The listing builds one solid part. Answer for the finished solid, in the listing's coordinates (mm). Round coordinates to 2 decimals unless told otherwise and drop trailing zeros. Write each loop counter-clockwise with the first axis right and the second up, starting at its lowest first coordinate (ties: lowest second). Pieces come first, ordered by that corner, then holes.
(1) The mould has two halves that part along Y. Classify faces 1 (the face through (21.403, 9.898, 1.479)), 2 (the face through (1, 2, 2)), 3 (the face through (73, 29, 2)): +Y half, -Y half, draft (parallel to the pull), parting line (faces both ways), or undercut.
(2) Each of these flat-tipped pins is pushed along its axis until it touches: pin 1 Ø9.5 at (x, y) = (16.4, 8.32) entering from +Z; pin 2 Ø4 at (x, y) = (23.5, 15) entering from -Z. Where does it stop, or does it pass through?
(3) Find the intervals of material crossed by probe 1 along X at (y, z) = (4.5, 2); probe 2 along X at (y, z) = (10.75, 2); probe 3 along Y at (x, z) = (46, 1.5), in increasing order.
(4) A cutting plane is placed at B-B, the plane x = 37.5. Give the vertices of the cut face in (y, z).
(5) A cutting plane is placed at C-C, the plane x = 19.5. Give the vertices of the cut face in (y, z), and give its area (3 significant figures).
(6) A cutting plane is placed at A-A, the plane y = 15. Give the vertices of the cut face in (x, z), and give its area (3 significant figures).
(7) A cutting plane is placed at D-D, the plane z = 1.35. Give the number of separate pieces and of enclosed holes in the cut face, and give its area (3 significant figures).
from build123d import *

# Parameters (mm, degrees)
SKETCH_W   = 75
SKETCH_H   = 30
SKETCH_R   = 5.25
SKETCH_R_2 = 1.6
PAD_DEPTH  = 3
FILLET_R   = 5


with BuildPart() as part:
    # Sketch → Pad (new body)
    with BuildSketch(Plane.XY):
        with Locations((37.5, 15)):
            Rectangle(SKETCH_W, SKETCH_H)
        with Locations((16.609054, 22.319043)):
            Circle(SKETCH_R, mode=Mode.SUBTRACT)
        with Locations((37.5, 15)):
            Circle(SKETCH_R_2, mode=Mode.SUBTRACT)
        with Locations((3.5, 15)):
            Circle(SKETCH_R_2, mode=Mode.SUBTRACT)
        with Locations((71.5, 15)):
            Circle(SKETCH_R_2, mode=Mode.SUBTRACT)
        with Locations((23.5, 15)):
            Circle(SKETCH_R_2, mode=Mode.SUBTRACT)
        with Locations((51.5, 15)):
            Circle(SKETCH_R_2, mode=Mode.SUBTRACT)
        with Locations((30.60743, 22.105806)):
            Circle(SKETCH_R, mode=Mode.SUBTRACT)
        with Locations((44.605806, 21.89257)):
            Circle(SKETCH_R, mode=Mode.SUBTRACT)
        with Locations((58.604182, 21.679333)):
            Circle(SKETCH_R, mode=Mode.SUBTRACT)
        with Locations((16.395818, 8.320667)):
            Circle(SKETCH_R, mode=Mode.SUBTRACT)
        with Locations((30.394194, 8.10743)):
            Circle(SKETCH_R, mode=Mode.SUBTRACT)
        with Locations((44.39257, 7.894194)):
            Circle(SKETCH_R, mode=Mode.SUBTRACT)
        with Locations((58.390946, 7.680957)):
            Circle(SKETCH_R, mode=Mode.SUBTRACT)
    extrude(amount=PAD_DEPTH)

    # Fillet
    fillet_edges = [part.edges().sort_by_distance(p)[0] for p in [
        (0, 0, 1.5),
        (75, 0, 1.5),
        (75, 30, 1.5),
        (0, 30, 1.5),
    ]]
    fillet(fillet_edges, radius=FILLET_R)


solid = part.part
Solutions:
1. face 1: undercut
1. face 2: -Y half
1. face 3: +Y half
2. pin 1: passes through
2. pin 2: stops at z = 0
3. probe 1: x = 0.03 to 12.8, 20 to 26.58, 34.21 to 40.39, 48.4 to 54.21, 62.57 to 74.97
3. probe 2: x = 0 to 11.74, 21.05 to 25.86, 34.93 to 39.99, 48.8 to 54.13, 62.65 to 75
3. probe 3: y = 0 to 2.9, 12.89 to 16.83, 26.95 to 30
4. outline: (0, 0) - (13.4, 0) - (13.4, 3) - (0, 3) - close; (16.6, 0) - (30, 0) - (30, 3) - (16.6, 3) - close
5. outline: (0, 0) - (4.09, 0) - (4.09, 3) - (0, 3) - close; (12.55, 0) - (17.94, 0) - (17.94, 3) - (12.55, 3) - close; (26.7, 0) - (30, 0) - (30, 3) - (26.7, 3) - close
5. area: 38.3 mm2
6. outline: (0, 0) - (1.9, 0) - (1.9, 3) - (0, 3) - close; (5.1, 0) - (21.9, 0) - (21.9, 3) - (5.1, 3) - close; (25.1, 0) - (35.9, 0) - (35.9, 3) - (25.1, 3) - close; (39.1, 0) - (49.9, 0) - (49.9, 3) - (39.1, 3) - close; (53.1, 0) - (69.9, 0) - (69.9, 3) - (53.1, 3) - close; (73.1, 0) - (75, 0) - (75, 3) - (73.1, 3) - close
6. area: 177 mm2
7. separate pieces: 1
7. enclosed holes: 13
7. area: 1,500 mm2
